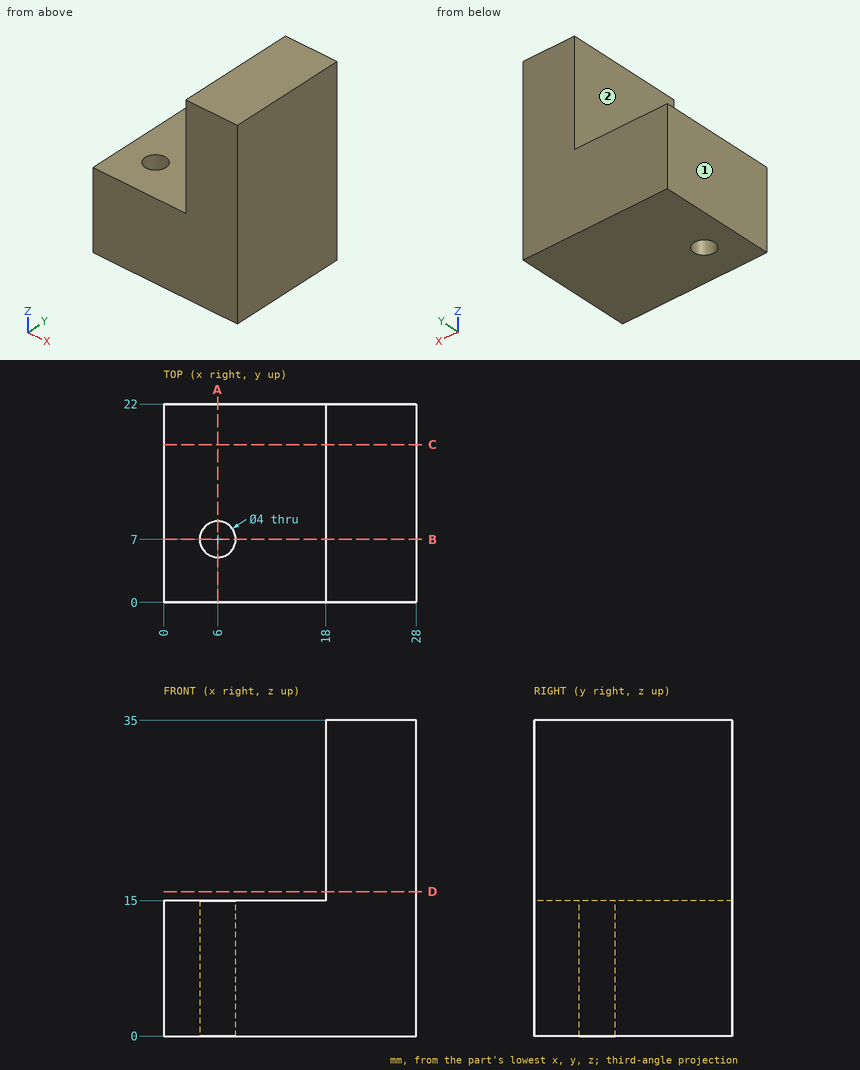
The drawing under review shows one solid part. Ordinate dimensions are in mm from its lowest x, y, z. A direction names the side the tool comes from. Round coordinates to 2 decimals unless told otherwise and drop trailing zeros. Order: outer loops, then holes, each group sorted by start corner. A loop starts at its lowest first (then second) coordinate and runs counter-clockwise, first axis right, second up. Notation, with made-up numbers: (27.5, -20) -> (44.5, -20) arc R19 cw to (44.5, -5) -> close; hole circle Ø10 at (-36.5, -5). An arc over 180 degrees is marked (long way). Use a Markdown table: item, result.
Item 1: For line 1 along Y through (x, z) = (6, 6.25); line 2 along X through (y, z) = (7, 7.5); line 3 along Z through (x, y) = (16.75, 5.75), list the stretches that pass through material, from the lowest coordinate up. Write a range as [from, to].
Resolved:
| item | result |
|---|---|
| line 1 | y = [0, 5], [9, 22] |
| line 2 | x = [0, 4], [8, 28] |
| line 3 | z = [0, 15] |
Item 2: Take a section at C-C (y = 17.5). State the section outline as (x, z) points.
Resolved:
| item | result |
|---|---|
| outline | (0, 0) -> (28, 0) -> (28, 35) -> (18, 35) -> (18, 15) -> (0, 15) -> close |
Item 3: Take a section at B-B (y = 7). State the section outline as (x, z) points.
Resolved:
| item | result |
|---|---|
| outline | (0, 0) -> (4, 0) -> (4, 15) -> (0, 15) -> close; (8, 0) -> (28, 0) -> (28, 35) -> (18, 35) -> (18, 15) -> (8, 15) -> close |
Item 4: Machinability: for the marked faces 1 and 2, which of the approach directions +Z, -Z, +X, -X, +Y, -Y give a long, thin tool a straight path to every point of the face, cutting with its end or side? Answer none if there is none.
Resolved:
| item | result |
|---|---|
| face 1 | +Z, -Z, -X, +Y, -Y |
| face 2 | +Z, -X, +Y, -Y |
Item 5: For pin 1 (1.5 mm diameter, centred on y = 11.5, z = 28.5, fed in from -X), flat-tipped, find the tip position at first contact; note if it passes through.
Resolved:
| item | result |
|---|---|
| pin 1 | stops at x = 18 |
Item 6: Take a section at D-D (z = 16). State the section outline as (x, y) points.
Resolved:
| item | result |
|---|---|
| outline | (18, 0) -> (28, 0) -> (28, 22) -> (18, 22) -> close |
Item 7: Take a section at A-A (x = 6). State the section outline as (y, z) points, plus the area to 3 significant figures.
Resolved:
| item | result |
|---|---|
| outline | (0, 0) -> (5, 0) -> (5, 15) -> (0, 15) -> close; (9, 0) -> (22, 0) -> (22, 15) -> (9, 15) -> close |
| area | 270 mm² |
